For this review, take the finished solid that the model builds, in its own axes (mm). A direction names the side the tool comes from. Round coordinates to 2 decimals unless told otherwise and drop trailing zeros. One line per question, with ' | ' between items. Start each with the question number.
1) Mouldability with a two-part tool opening along X and no side actions: class faces 3 (the face through (26.07, 3.5, -0.2)), 4 (the face through (3.123, 9.225, 6.025)), 5 (the face through (-5, 5, -10)) as pulls with the +X half, pulls with the -X half, needs draft (parallel to the pull), parting line crosses it, or undercut.
2) For faces 1 (the face through (-18.61, 2.47, -13.39)), 2 (the face through (-3.123, 9.225, -6.025)), list the 3-axis set-ups (+Z, -Z, +X, -X, +Y, -Y) from which the entire face can be reached by the end or side of a thin tool; tool diameter is ignored.
3) For pin 1 Ø2 at (x, z) = (1, 8) entering from +Y; pin 2 Ø5 at (x, y) = (-3, 1) entering from -Z; pin 3 Ø4 at (y, z) = (10, -10.5) entering from -X; pin 4 Ø5 at (y, z) = (9.5, -5) entering from -X, all flat-tipped, find the tip position at first contact; note any pin that passes through.
4) For probe 1 along X at (y, z) = (7.5, 0); probe 2 along Z at (x, y) = (-20, 3.95); probe 3 along X at (y, z) = (3.75, -14), list the stretches that pass through material, from the lowest coordinate up. Write a range as from..to.
5) We need section A-A (z = 12.5). State how many separate pieces and enclosed holes the cut face has, and give its area (3 significant figures).
```python
from build123d import *

# Parameters (mm, degrees)
SKETCH_1_W          = 55
SKETCH_1_H          = 38
EXTRUDE_1_DEPTH     = 5
SKETCH_2_R          = 10.9
EXTRUDE_2_DEPTH     = 6
SKETCH_3_R          = 4
CUT_EXTRUDE_1_DEPTH = 36.18877662
CUT_EXTRUDE_2_DEPTH = 3.6
SKETCH_5_R          = 0.5
CUT_EXTRUDE_3_DEPTH = 4
FILLET_1_R          = 5
FILLET_2_R          = 5
FILLET_3_R          = 5
FILLET_4_R          = 5
FILLET_5_R          = 5
SKETCH_6_R          = 1.65
CUT_EXTRUDE_4_DEPTH = 36.18877662


with BuildPart() as part:
    # 草图1 → 凸台-拉伸1 (new body)
    with BuildSketch(Plane(origin=(0, 0, 0), x_dir=(1, 0, 0), z_dir=(0, 1, 0))):
        Rectangle(SKETCH_1_W, SKETCH_1_H)
    extrude(amount=EXTRUDE_1_DEPTH)

    # 草图2 → 凸台-拉伸2 (add)
    with BuildSketch(Plane(origin=(0, 5, 0), x_dir=(1, 0, 0), z_dir=(0, 1, 0))):
        with Locations(Location((0, 0, 0), (0, 0, 270))):
            Circle(SKETCH_2_R)
    extrude(amount=EXTRUDE_2_DEPTH)

    # 草图3 → 切除-拉伸1 (cut, through all)
    with BuildSketch(Plane.XZ):
        with Locations(Location((0, 0, 0), (0, 0, 270))):
            Circle(SKETCH_3_R)
    extrude(amount=-CUT_EXTRUDE_1_DEPTH, mode=Mode.SUBTRACT)

    # 草图4 → 切除-拉伸2 (cut)
    with BuildSketch(Plane(origin=(0, 11, 0), x_dir=(1, 0, 0), z_dir=(0, 1, 0))):
        Polygon((3.674809939, -1.579801226), (2.341337155, -12.320336373), (-2.341337155, -12.320336373), (-3.674809939, -1.579801226), align=None)
        Polygon((-3.674809939, 1.579801226), (-2.341337155, 12.320336373), (2.341337155, 12.320336373), (3.674809939, 1.579801226), align=None)
    extrude(amount=-CUT_EXTRUDE_2_DEPTH, mode=Mode.SUBTRACT)

    # 草图5 → 切除-拉伸3 (cut)
    with BuildSketch(Plane(origin=(0, 7.4, 0), x_dir=(1, 0, 0), z_dir=(0, 1, 0))):
        with Locations(Location((0, -6.5, 0), (0, 0, 270))):
            Circle(SKETCH_5_R)
        with Locations(Location((0, 6.5, 0), (0, 0, 270))):
            Circle(SKETCH_5_R)
    extrude(amount=-CUT_EXTRUDE_3_DEPTH, mode=Mode.SUBTRACT)

    # 圆角1
    fillet_1_edges = [part.edges().sort_by_distance(p)[0] for p in [
        (27.5, 2.5, 19),
    ]]
    fillet(fillet_1_edges, radius=FILLET_1_R)

    # 圆角2
    fillet_2_edges = [part.edges().sort_by_distance(p)[0] for p in [
        (-27.5, 2.5, 19),
    ]]
    fillet(fillet_2_edges, radius=FILLET_2_R)

    # 圆角3
    fillet_3_edges = [part.edges().sort_by_distance(p)[0] for p in [
        (-27.5, 2.5, -19),
    ]]
    fillet(fillet_3_edges, radius=FILLET_3_R)

    # 圆角4
    fillet_4_edges = [part.edges().sort_by_distance(p)[0] for p in [
        (27.5, 2.5, -19),
    ]]
    fillet(fillet_4_edges, radius=FILLET_4_R)

    # 圆角5
    fillet_5_edges = [part.edges().sort_by_distance(p)[0] for p in [
        (27.5, 5, 0),
        (0, 5, 19),
        (-27.5, 5, 0),
        (0, 5, -19),
        (26.035533906, 5, 17.535533906),
        (-26.035533906, 5, 17.535533906),
        (-26.035533906, 5, -17.535533906),
        (26.035533906, 5, -17.535533906),
    ]]
    fillet(fillet_5_edges, radius=FILLET_5_R - 0.0001)  # a hair under: the kernel refuses the full size

    # 草图6 → 切除-拉伸4 (cut, through all)
    with BuildSketch(Plane.XZ):
        with Locations(Location((-20, 12.5, 0), (0, 0, 270))):
            Circle(SKETCH_6_R)
        with Locations(Location((20, 12.5, 0), (0, 0, 270))):
            Circle(SKETCH_6_R)
        with Locations(Location((20, -12.5, 0), (0, 0, 270))):
            Circle(SKETCH_6_R)
        with Locations(Location((-20, -12.5, 0), (0, 0, 270))):
            Circle(SKETCH_6_R)
    extrude(amount=-CUT_EXTRUDE_4_DEPTH, mode=Mode.SUBTRACT)


solid = part.part
```
Answers below:
1) face 3: pulls with the +X half | face 4: undercut | face 5: needs draft
2) face 1: +Y, -Y | face 2: +Y
3) pin 1: y = 7.4 | pin 2: z = -19 | pin 3: x = -6.82 | pin 4: x = -10.61
4) probe 1: -10.9..-4, 4..10.9 | probe 2: -17.07..-14.15, -10.85..10.85, 14.15..17.07 | probe 3: -25.81..-20.69, -19.31..19.31, 20.69..25.81
5) separate pieces: 3 | enclosed holes: 0 | area: 231 mm^2
